Check sheet for the modelled part. Datum: model origin and axes. Units: mm. A direction names the side the tool comes from. Give positions to 0.01 mm unless a question says otherwise; leave off trailing zeros. Order: outer loops, then holes, each group sorted by start corner. A loop starts at its lowest first (then second) coordinate and runs counter-clockwise, first axis right, second up.
Item 1: Material ranges on line 1 along Z through (x, y) = (1.5, 16); line 2 along Y through (x, z) = (-18, -2); line 3 along X through (y, z) = (2.75, 13), recorded low to high.
Item 2: Sectioned sample at B-B on z = 3. Record the boundary of the cut face in (x, y).
Item 3: Release check for a two-part mould opening along X. For faces 1 (the cylindrical face through (17.74, 0.84, 12.22)), 2 (the flat face through (0, 1, 16.828)), 3 (the flat face through (2.934, 9, 6)), 4 (the cylindrical face through (-18.063, 0.838, -12.728)) record: released by +X, released by -X, zero draft, split by the parting line, or undercut.
Item 4: Access from +Z, -Z, +X, -X, +Y, -Y to the whole of each face (thin tool, end or side, straight path). Record for faces 5 (the flat face through (-7, 9, -1.838)), 6 (the flat face through (-6, 9, 13.482)), 7 (the flat face through (-15.856, 9, 6)), 8 (the flat face through (0, 1, -16.828)).
Item 5: Sectioned sample at C-C on z = 14.5. Record the boundary of the cut face in (x, y), and give its area (3 significant figures).
Item 6: Sectioned sample at A-A on x = 2. Record the boundary of the cut face in (y, z), and give its area (3 significant figures).
Item 7: Gauge pin test, flat ends, axial feed: P1, Ø4, axis at x = 0, z = -11, coming from the +Y side; P2, Ø7.5, axis at y = 11, z = 8.5, coming from the -X side; P3, Ø4, axis at x = -4, y = 10, coming from the +Z side. Record the tip position at first contact, or that the pin passes through.
Item 8: Sectioned sample at D-D on y = 15. Record the boundary of the cut face in (x, z).
Autodesk Inventor part; units mm, degrees
ref_plane "YZ Plane" through (0, 0, 0) normal (1, 0, 0) x (0, 1, 0)
ref_plane "XZ Plane" through (0, 0, 0) normal (0, 1, 0) x (-1, 0, 0)
ref_plane "XY Plane" through (0, 0, 0) normal (0, 0, 1) x (1, 0, 0)
sketch "Sketch1" plane through (0, 0, 0) normal (0, 1, 0) x (-1, 0, 0)
  line L0 (19.8755, 16.8275) -> (-19.8755, 16.8275)
  line L1 (-19.8755, 16.8275) -> (-19.8755, -16.8275)
  line L2 (-19.8755, -16.8275) -> (19.8755, -16.8275)
  line L3 (19.8755, -16.8275) -> (19.8755, 16.8275)
  line L4 (19.8755, 16.8275) -> (-19.8755, -16.8275) construction
  line L5 (-19.8755, 16.8275) -> (19.8755, -16.8275) construction
  circle A0 centre (16.4465, -13.3985) radius 1.75
  circle A1 centre (-16.4465, 13.3985) radius 1.75
  line L6 (15.8555, -1.8383) -> (-2.9345, -1.8383)
  line L7 (-2.9345, -1.8383) -> (-2.9345, 13.4817)
  line L8 (-2.9345, 13.4817) -> (15.8555, 13.4817)
  line L9 (15.8555, 13.4817) -> (15.8555, -1.8383)
  point P0 (0, 0)
  dimension "d0" = 39.751
  dimension "d1" = 33.655
  dimension "d2" = 3.5
  dimension "d3" = 3.5
  dimension "d4" = 3.429
  dimension "d5" = 3.429
  dimension "d6" = 3.429
  dimension "d7" = 3.429
  dimension "d8" = 18.79
  dimension "d9" = 15.32
  dimension "d10" = 24.2439
  dimension "d11" = 24.2439
extrude "Extrusion1" add sketch "Sketch1" along normal blind 1.7
extrude "Extrusion2" add sketch "Sketch1" along normal blind 17.44 contours L6 L7 L8 L9
sketch "Sketch2" plane through (0, 1.7, 0) normal (0, 1, 0) x (1, 0, 0)
  line L0 (-18.4674, 8.6665) -> (19.4938, 8.6665) construction
  line L1 (19.4938, 8.6665) -> (19.4938, 5.0304) construction
  line L2 (19.4938, 5.0304) -> (-18.4674, 5.0304) construction
  line L3 (-18.4674, 5.0304) -> (-18.4674, 8.6665) construction
  point P0 (0, 0)
properties part number "Driver Kipas v2"
Report:
1. line 1: z = -1.84 to 13.48
1. line 2: y = 0 to 1.7
1. line 3: x = -15.86 to 2.93
2. outline: (-19.88, 0) - (19.88, 0) - (19.88, 1.7) - (2.93, 1.7) - (2.93, 17.44) - (-15.86, 17.44) - (-15.86, 1.7) - (-19.88, 1.7) - close
3. face 1: undercut
3. face 2: zero draft
3. face 3: released by +X
3. face 4: undercut
4. face 5: -Z, +X, -X, +Y
4. face 6: +Z, +X, -X, +Y
4. face 7: +Z, -Z, -X, +Y
4. face 8: -Z, +X, -X, +Y, -Y
5. outline: (-19.88, 0) - (15.09, 0) - (15.09, 1.7) - (-19.88, 1.7) - close; (17.81, 0) - (19.88, 0) - (19.88, 1.7) - (17.81, 1.7) - close
5. area: 63.0 mm2
6. outline: (0, -16.83) - (1.7, -16.83) - (1.7, -1.84) - (17.44, -1.84) - (17.44, 13.48) - (1.7, 13.48) - (1.7, 16.83) - (0, 16.83) - close
6. area: 298 mm2
7. P1: stops at y = 1.7
7. P2: stops at x = -15.86
7. P3: stops at z = 13.48
8. outline: (-15.86, -1.84) - (2.93, -1.84) - (2.93, 13.48) - (-15.86, 13.48) - close
